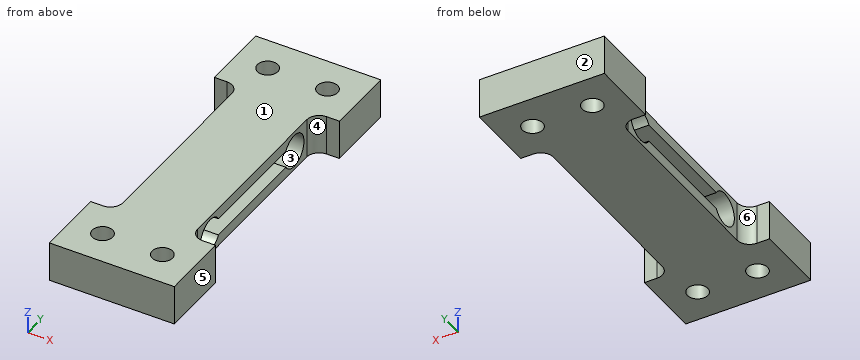
from build123d import *

# Parameters (mm, degrees)
SKETCH1_W                = 12.538434267
SKETCH1_H                = 35
BOSS_EXTRUDE1_DEPTH      = 4
SKETCH2_W                = 2.5
SKETCH2_H                = 21
CUT_EXTRUDE1_DEPTH       = 5
SKETCH3_W                = 2.538434267
SKETCH3_H                = 21
CUT_EXTRUDE2_DEPTH       = 5
CUT_EXTRUDE3_DEPTH       = 11.038434267
SKETCH5_W                = 7.5
SKETCH5_H                = 1.65
SKETCH6_W                = 7.5
SKETCH6_H                = 1.65
M2_5X0_45_TAPPED_HOLE1_D = 2.05
FILLET1_R                = 1.25


with BuildPart() as part:
    # Sketch1 → Boss-Extrude1 (new body)
    with BuildSketch(Plane.XY.offset(4)):
        with Locations((-3.730782867, 17.5)):
            Rectangle(SKETCH1_W, SKETCH1_H)
    extrude(amount=-BOSS_EXTRUDE1_DEPTH)

    # Sketch2 → Cut-Extrude1 (cut, through all)
    with BuildSketch(Plane(origin=(0, 0, 0), x_dir=(-1, 0, 0), z_dir=(0, 0, -1))):
        with Locations((8.75, 17.5)):
            Rectangle(SKETCH2_W, SKETCH2_H)
    extrude(amount=-CUT_EXTRUDE1_DEPTH, mode=Mode.SUBTRACT)

    # Sketch3 → Cut-Extrude2 (cut, through all)
    with BuildSketch(Plane(origin=(0, 0, 0), x_dir=(-1, 0, 0), z_dir=(0, 0, -1))):
        with Locations((-1.269217133, 17.5)):
            Rectangle(SKETCH3_W, SKETCH3_H)
    extrude(amount=-CUT_EXTRUDE2_DEPTH, mode=Mode.SUBTRACT)

    # Sketch4 → Cut-Extrude3 (cut, through all)
    with BuildSketch(Plane.ZY.offset(7.5)):
        with BuildLine():
            Line((2.855933763, 11.78563014), (2.855933763, 23.21436986))
            ThreePointArc((2.855933763, 23.21436986), (1.992824856, 22.975015601), (1.13183027, 23.221867319))
            Line((1.13183027, 23.221867319), (1.13183027, 11.778132681))
            ThreePointArc((1.13183027, 11.778132681), (1.992824856, 12.024984399), (2.855933763, 11.78563014))
        make_face()
    extrude(amount=-CUT_EXTRUDE3_DEPTH, mode=Mode.SUBTRACT)

    # Sketch5 → Cut-Revolve1 (revolve, cut)
    with BuildSketch(Plane(origin=(0, 0, 2), x_dir=(-1, 0, 0), z_dir=(0, 0, -1))):
        with Locations((3.75, 25.45)):
            Rectangle(SKETCH5_W, SKETCH5_H)
    revolve(axis=Axis((0, 24.625, 2), (-1, 0, 0)), mode=Mode.SUBTRACT)

    # Sketch6 → Cut-Revolve2 (revolve, cut)
    with BuildSketch(Plane(origin=(0, 0, 2), x_dir=(-1, 0, 0), z_dir=(0, 0, -1))):
        with Locations((3.75, 11.2)):
            Rectangle(SKETCH6_W, SKETCH6_H)
    revolve(axis=Axis((0, 10.375, 2), (-1, 0, 0)), mode=Mode.SUBTRACT)

    # M2.5x0.45 Tapped Hole1 (through all)
    with Locations(Plane.XY.offset(4)):
        with Locations((-0.730782866, 3.5), (-6.730782866, 3.5), (-0.730782866, 31.5), (-6.730782866, 31.5)):
            Hole(M2_5X0_45_TAPPED_HOLE1_D / 2)

    # Fillet1
    fillet1_edges = [part.edges().sort_by_distance(p)[0] for p in [
        (-7.5, 7, 2),
        (-7.5, 28, 2),
        (0, 28, 2),
        (0, 7, 2),
    ]]
    fillet(fillet1_edges, radius=FILLET1_R)


solid = part.part
Geometry: final body of the model. Coordinates: model frame, mm. Face numbers are marked on the shaded views. A direction names the side the tool comes from. Give positions to 0.01 mm unless a question says otherwise; leave off trailing zeros. Loops run counter-clockwise (first coordinate to the right, second up) from the corner with the lowest first, then second, coordinate; pieces in that order, holes last. Notation, with made-up numbers: (56, 3.5) - (93, 3.5) arc R20 cw to (93, 36.5) - close; hole circle Ø1 at (51, 86.25). An arc over 180 degrees is marked (long way). One line per question, with ' | ' between items. Start each with the question number.
(1) Section query D-D on x = -6.5. Return loops of the section in (y, z) (3 decimals).
(2) Section query A-A on y = 3.5. Return loops of the section in (x, z), then the cut area to 3 significant figures.
(3) Section query C-C on y = 18. Return loops of the section in (x, z).
(4) Contact query for flat-ended pins moving along their axis: pin 1 (3.5 mm diameter, centred on x = -6.73, y = 3.5, fed in from -Z); pin 2 (1.2 mm diameter, centred on y = 20, z = 1.5, fed in from +X); pin 3 (2 mm diameter, centred on y = 18.5, z = 1.5, fed in from -X). Output: stop coordinate, or through.
(5) Reachability of the marked faces 5 and 6 from +Z, -Z, +X, -X, +Y, -Y: full face, straight path, thin tool, end or side. Return the list, or none.
(6) Pull-direction query (Y, two-part tool) for the marked faces 1, 2, 3 and 4; classes: released by +Y, released by -Y, zero draft, split by the parting line, or undercut.
(7) Ray query, line 1 (Z direction, x = -0.5, y = 18); line 2 (Y direction, x = -0.25, z = 2) (3 decimals); line 3 (Y direction, x = -9, z = 2.15). Return the intervals inside material, ascending. Write a range as from..to.
(8) Section query B-B on z = 2. Return loops of the section in (x, y) (3 decimals), then the cut area to 3 significant figures.
The answers:
1) outline: (0, 0) - (2.501, 0) - (2.501, 4) - (0, 4) - close; (4.499, 0) - (30.501, 0) - (30.501, 4) - (4.499, 4) - close; (32.499, 0) - (35, 0) - (35, 4) - (32.499, 4) - close; hole (11.778, 1.132) - (23.222, 1.132) arc R1.65 ccw (long way) to (23.214, 2.856) - (11.786, 2.856) arc R1.65 ccw (long way) to start
2) outline: (-10, 0) - (-7.76, 0) - (-7.76, 4) - (-10, 4) - close; (-5.71, 0) - (-1.76, 0) - (-1.76, 4) - (-5.71, 4) - close; (0.29, 0) - (2.54, 0) - (2.54, 4) - (0.29, 4) - close | area: 33.8 mm2
3) outline: (-7.5, 0) - (0, 0) - (0, 1.13) - (-7.5, 1.13) - close; (-7.5, 2.86) - (0, 2.86) - (0, 4) - (-7.5, 4) - close
4) pin 1: z = 0 | pin 2: x = 0 | pin 3: x = -7.5
5) face 5: +Z, -Z, +X, +Y, -Y | face 6: +Z, -Z, -X
6) face 1: zero draft | face 2: released by +Y | face 3: undercut | face 4: undercut
7) line 1: 0..1.13, 2.86..4 | line 2: 0..2.595, 4.405..8.725, 26.275..30.595, 32.405..35 | line 3: 0..7, 28..35
8) outline: (-10, 0) - (2.538, 0) - (2.538, 7) - (1.25, 7) arc R1.25 cw to (0, 8.25) - (0, 8.725) - (-7.5, 8.725) - (-7.5, 8.25) arc R1.25 cw to (-8.75, 7) - (-10, 7) - close; (-10, 28) - (-8.75, 28) arc R1.25 cw to (-7.5, 26.75) - (-7.5, 26.275) - (0, 26.275) - (0, 26.75) arc R1.25 cw to (1.25, 28) - (2.538, 28) - (2.538, 35) - (-10, 35) - close; hole circle Ø2.05 at (-6.731, 3.5); hole circle Ø2.05 at (-6.731, 31.5); hole circle Ø2.05 at (-0.731, 3.5); hole circle Ø2.05 at (-0.731, 31.5) | area: 190 mm2
